Geometry check sheet. Reference: the model listing, model coordinates, mm. A direction names the side the tool comes from. Give positions to 0.01 mm unless a question says otherwise; leave off trailing zeros. Loops run counter-clockwise (first coordinate to the right, second up) from the corner with the lowest first, then second, coordinate; pieces in that order, holes last. Notation, with made-up numbers: (87, 87.5) -> (105, 87.5) arc R25 cw to (105, 100.5) -> close; hole circle Ø9 at (-29.75, 10). An arc over 180 degrees is marked (long way). One line per question, with ' | ' between items.
from build123d import *

# Parameters (mm, degrees)
SKETCH1_W           = 305
SKETCH1_H           = 125
SKETCH1_R           = 3
BOSS_EXTRUDE1_DEPTH = 10
SKETCH7_W           = 40
SKETCH7_H           = 50
SKETCH7_H_2         = 15
BOSS_EXTRUDE2_DEPTH = 22.639320225
BOSS_EXTRUDE3_REACH = 324.786
SKETCH11_R          = 30
SKETCH11_R_2        = 13
SKETCH12_W          = 35.5
SKETCH12_H          = 75
CUT_EXTRUDE2_DEPTH  = 341.404171537
CUT_EXTRUDE1_DEPTH  = 2
SKETCH16_R          = 1.55
CUT_EXTRUDE3_DEPTH  = 339.045854878
FILLET3_R           = 10
CHAMFER2_SIZE       = 1.65


with BuildPart() as part:
    # Sketch1 → Boss-Extrude1 (new body)
    with BuildSketch(Plane(origin=(0, 0, 0), x_dir=(1, 0, 0), z_dir=(0, 1, 0))):
        with Locations((152.5, 62.5)):
            Rectangle(SKETCH1_W, SKETCH1_H)
        with Locations(Location((280, 25, 0), (0, 0, 270))):
            Circle(SKETCH1_R, mode=Mode.SUBTRACT)
        with Locations(Location((25, 25, 0), (0, 0, 90))):
            Circle(SKETCH1_R, mode=Mode.SUBTRACT)
        with Locations(Location((107.5, 115, 0), (0, 0, 270))):
            Circle(SKETCH1_R, mode=Mode.SUBTRACT)
        with Locations(Location((107.5, 95, 0), (0, 0, 270))):
            Circle(SKETCH1_R, mode=Mode.SUBTRACT)
        with Locations(Location((197.5, 115, 0), (0, 0, 90))):
            Circle(SKETCH1_R, mode=Mode.SUBTRACT)
        with Locations(Location((197.5, 95, 0), (0, 0, 90))):
            Circle(SKETCH1_R, mode=Mode.SUBTRACT)
    extrude(amount=BOSS_EXTRUDE1_DEPTH)

    # Sketch7 → Boss-Extrude2 (add)
    with BuildSketch(Plane(origin=(0, 10, 0), x_dir=(1, 0, 0), z_dir=(0, 1, 0))):
        with Locations((152.5, 49.5)):
            Rectangle(SKETCH7_W, SKETCH7_H)
        with Locations((152.5, 117.5)):
            Rectangle(SKETCH7_W, SKETCH7_H_2)
    extrude(amount=BOSS_EXTRUDE2_DEPTH)

    # Boss-Extrude3: up to this face of the body (flat: up to its plane)
    boss_extrude3_end = Plane(part.part.faces().sort_by_distance((152.5, 8.736156851, -125))[0])
    # Sketch11 → Boss-Extrude3 (add, up to the picked face)
    with BuildSketch(Plane.XY.offset(-24.5), mode=Mode.PRIVATE) as boss_extrude3_sk1:
        with Locations(Location((152.5, 55, 0), (0, 0, 311.810314896))):
            Circle(SKETCH11_R)
        with Locations((152.5, 55)):
            Circle(SKETCH11_R_2, mode=Mode.SUBTRACT)
    boss_extrude3_tool1 = split(extrude(boss_extrude3_sk1.sketch, amount=-BOSS_EXTRUDE3_REACH, mode=Mode.PRIVATE), bisect_by=boss_extrude3_end, keep=Keep.BOTH, mode=Mode.PRIVATE)
    add(boss_extrude3_tool1.solids().sort_by(Axis((133.065685, 76.728224, -24.5), (0, 0, -1)))[0])

    # Sketch12 → Cut-Extrude2 (cut, through all)
    with BuildSketch(Plane(origin=(305, 0, 0), x_dir=(0, 0, -1), z_dir=(1, 0, 0))):
        with Locations((92.25, 47.5)):
            Rectangle(SKETCH12_W, SKETCH12_H)
    extrude(amount=-CUT_EXTRUDE2_DEPTH, mode=Mode.SUBTRACT)

    # Sketch6 → Cut-Extrude1 (cut)
    with BuildSketch(Plane(origin=(0, 10, 0), x_dir=(1, 0, 0), z_dir=(0, 1, 0))):
        Polygon((27.886751346, 30), (30.773502692, 25), (27.886751346, 20), (22.113248654, 20), (19.226497308, 25), (22.113248654, 30), align=None)
        Polygon((274.226497308, 25), (277.113248654, 20), (282.886751346, 20), (285.773502692, 25), (282.886751346, 30), (277.113248654, 30), align=None)
    extrude(amount=-CUT_EXTRUDE1_DEPTH, mode=Mode.SUBTRACT)

    # Sketch16 → Cut-Extrude3 (cut, through all)
    with BuildSketch(Plane(origin=(0, 10, 0), x_dir=(1, 0, 0), z_dir=(0, 1, 0))):
        with Locations(Location((16, 7.5, 0), (0, 0, 270))):
            Circle(SKETCH16_R)
        with Locations(Location((98.95, 7.5, 0), (0, 0, 270))):
            Circle(SKETCH16_R)
        with Locations(Location((16, 55.866, 0), (0, 0, 270))):
            Circle(SKETCH16_R)
        with Locations(Location((91.33, 55.866, 0), (0, 0, 270))):
            Circle(SKETCH16_R)
    extrude(amount=-CUT_EXTRUDE3_DEPTH, mode=Mode.SUBTRACT)

    # Fillet3
    fillet3_edges = [part.edges().sort_by_distance(p)[0] for p in [
        (305, 5, 0),
        (0, 5, 0),
    ]]
    fillet(fillet3_edges, radius=FILLET3_R)

    # Chamfer2
    chamfer2_edges = [part.edges().sort_by_distance(p)[0] for p in [
        (98.95, 0, -9.05),
        (16, 0, -57.416),
        (91.33, 0, -57.416),
        (16, 0, -9.05),
    ]]
    chamfer(chamfer2_edges, length=CHAMFER2_SIZE)


solid = part.part
Item 1: Sectioned sample at B-B (x = 280). Record the cut outline in (y, z).
Result:
outline: (0, -125) -> (10, -125) -> (10, -30) -> (8, -30) -> (8, -28) -> (0, -28) -> close; (0, -22) -> (8, -22) -> (8, -20) -> (10, -20) -> (10, 0) -> (0, 0) -> close
Item 2: Set-up check for faces 5 (the face through (22.5, 8, -22.8)), 6 (the face through (152, 39, -24.5)), 7 (the face through (105.7, 4.9, -97.4)), 8 (the face through (152, 39, -110)), 9 (the face through (99, 1.5, -9.2)): record each of +Z, -Z, +X, -X, +Y, -Y from which the full face is reachable in a straight line by a thin tool's end or side.
Result:
face 5: +Y | face 6: +Z, +X, -X, +Y | face 7: +Y, -Y | face 8: +X, -X, +Y | face 9: -Y
Item 3: Sectioned sample at D-D (z = -95). Record the cut outline in (x, y), plus the area to 3 significant figures.
Result:
outline: (0, 0) -> (104.5, 0) -> (104.5, 10) -> (0, 10) -> close; (110.5, 0) -> (194.5, 0) -> (194.5, 10) -> (110.5, 10) -> close; (200.5, 0) -> (305, 0) -> (305, 10) -> (200.5, 10) -> close | area: 2,930 mm2
Item 4: Sectioned sample at C-C (x = 152.5). Record the cut outline in (y, z).
Result:
outline: (0, -125) -> (42, -125) -> (42, -110) -> (10, -110) -> (10, -74.5) -> (42, -74.5) -> (42, -24.5) -> (10, -24.5) -> (10, 0) -> (0, 0) -> close; (68, -125) -> (85, -125) -> (85, -110) -> (68, -110) -> close; (68, -74.5) -> (85, -74.5) -> (85, -24.5) -> (68, -24.5) -> close
Item 5: Sectioned sample at A-A (z = -115). Record the cut outline in (x, y), plus the area to 3 significant figures.
Result:
outline: (0, 0) -> (104.5, 0) -> (104.5, 10) -> (0, 10) -> close; (110.5, 0) -> (194.5, 0) -> (194.5, 10) -> (172.5, 10) -> (172.5, 32.64) arc R30 ccw (long way) to (132.5, 32.64) -> (132.5, 10) -> (110.5, 10) -> close; (200.5, 0) -> (305, 0) -> (305, 10) -> (200.5, 10) -> close; hole circle Ø26 at (152.5, 55) | area: 5,920 mm2
Item 6: Depth check by flat-ended pin: pin 1 Ø12 at (y, z) = (74.5, -28) entering from -X; pin 2 Ø10 at (x, z) = (242, -90.5) entering from +Y; pin 3 Ø5 at (x, z) = (277.5, -24.5) entering from +Y. Enter the tip coordinate at first touch or a pass-through.
Result:
pin 1: x = 125.71 | pin 2: y = 10 | pin 3: y = 8
Item 7: Release check for a two-part mould opening along X. For faces 1 (the face through (153.513, 84.983, -117.395)), 2 (the face through (151, 5, 0)), 3 (the face through (172.5, 21, -117)), 4 (the face through (282.5, 8, -22.8)) record: pulls with the +X half, pulls with the -X half, needs draft (parallel to the pull), parting line crosses it, or undercut.
Result:
face 1: parting line crosses it | face 2: needs draft | face 3: pulls with the +X half | face 4: undercut
Item 8: Scan lines: probe 1 along Z at (x, y) = (197.5, 5.75); probe 2 along X at (y, z) = (5, -95); probe 3 along Z at (x, y) = (280, 4). Record each from-to range of solid material in increasing order.
Result:
probe 1: -125 to -118, -112 to -98, -92 to 0 | probe 2: 0 to 104.5, 110.5 to 194.5, 200.5 to 305 | probe 3: -125 to -28, -22 to 0
